For this review, take the finished solid that the model builds, in its own axes (mm). A direction names the side the tool comes from. Round coordinates to 2 decimals unless told otherwise and drop trailing zeros. Write each loop counter-clockwise with the first axis right and the second up, starting at its lowest first coordinate (ties: lowest second). Pieces come first, ordered by that corner, then holes. Notation, with made-up numbers: (42.25, -0.75) -> (64.25, -0.75) arc R11 ccw to (64.25, 8.25) -> close; hole circle Ø6 at (-6.5, 44). An arc over 180 degrees is marked (long way). Answer as CSV lines item,"result". Start each with the question number.
Item 1: Wall thickness on probe 1 along Y at (x, z) = (-20, -30); probe 2 along X at (y, z) = (-32.5, -11.5); probe 3 along Z at (x, y) = (-17.5, -6.5): over which ranges is each line inside the solid? List them lowest first. Write a range as from..to.
Item 2: Take a section at C-C on y = -14.5. Give the boundary of the cut face in (x, z), then the cut area to 3 significant figures.
Item 3: Take a section at B-B on z = 0. Give the boundary of the cut face in (x, y).
Item 4: Take a section at A-A on x = 0. Give the boundary of the cut face in (y, z).
Item 5: Machinability: for faces 1 (the cylindrical face through (-15.12, -28.84, -11.59)), 2 (the flat face through (-2, 0, 2)), which of the approach directions +Z, -Z, +X, -X, +Y, -Y give a long, thin tool a straight path to every point of the face, cutting with its end or side? Answer none if there is none.
Item 6: Take a section at D-D on x = 83. Give the boundary of the cut face in (y, z).
Item 7: For pin 1 Ø1 at (x, z) = (-87.5, 37.5) entering from +Y; pin 2 Ø6 at (x, z) = (-77, 96.5) entering from -Y, all flat-tipped, find the tip position at first contact; note any pin that passes through.
```python
from build123d import *

# Parameters (mm, degrees)
F0_R     = 19.05
F1_DEPTH = 53.594
F0_R_2   = 152.4
F2_DEPTH = 4.7625
F0_W     = 457.2
F0_H     = 355.6
F3_DEPTH = 15.875


with BuildPart() as f1:
    # F0 (on Front) → F1 (new body)
    with BuildSketch(Plane.XZ):
        Circle(F0_R)
    extrude(amount=F1_DEPTH)

    # F0 (on Front) → F2 (join)
    with BuildSketch(Plane.XZ):
        Circle(F0_R_2)
        Circle(F0_R, mode=Mode.SUBTRACT)
    extrude(amount=F2_DEPTH)


with BuildPart() as f3:
    # F0 (on Front) → F3 (new body)
    with BuildSketch(Plane.XZ):
        Rectangle(F0_W, F0_H)
        Circle(F0_R_2, mode=Mode.SUBTRACT)
    extrude(amount=F3_DEPTH)


solid = f1.part
```
Output values:
1,probe 1,"y = -4.76..0"
1,probe 2,"x = -15.19..15.19"
1,probe 3,"z = -7.53..7.53"
2,outline,"circle Ø38.1 at (0, 0)"
2,area,"1,140 mm^2"
3,outline,"(-152.4, -4.76) -> (-19.05, -4.76) -> (-19.05, -53.59) -> (19.05, -53.59) -> (19.05, -4.76) -> (152.4, -4.76) -> (152.4, 0) -> (-152.4, 0) -> close"
4,outline,"(-53.59, -19.05) -> (-4.76, -19.05) -> (-4.76, -152.4) -> (0, -152.4) -> (0, 152.4) -> (-4.76, 152.4) -> (-4.76, 19.05) -> (-53.59, 19.05) -> close"
5,face 1,"-Y"
5,face 2,"+Z, -Z, +X, -X, +Y"
6,outline,"(-4.76, -127.82) -> (0, -127.82) -> (0, 127.82) -> (-4.76, 127.82) -> close"
7,pin 1,"stops at y = 0"
7,pin 2,"stops at y = -4.76"
